Here's how the part is built. I have some questions about the finished solid (model axes, mm). A direction names the side the tool comes from. Give positions to 0.01 mm unless a question says otherwise; leave off trailing zeros. Order: outer loops, then holes, each group sorted by start corner. A loop starts at its lowest first (then second) coordinate and runs counter-clockwise, first axis right, second up.
from build123d import *

# Parameters (mm, degrees)
PAD_DEPTH    = 16
POCKET_DEPTH = 1


with BuildPart() as part:
    # Sketch → Pad (new body)
    with BuildSketch(Plane.XY):
        Polygon((0, 413.879036), (0, 490), (460, 490), (460, 0), (0, 0), align=None)
    extrude(amount=-PAD_DEPTH)

    # Sketch002 (on Face7 of Pad) → Pocket (cut)
    with BuildSketch(Plane(origin=(0, 0, -16), x_dir=(1, 0, 0), z_dir=(0, 0, -1))):
        Polygon((0, 0), (0, -71.973152), (460, 0), align=None)
    extrude(amount=-POCKET_DEPTH, mode=Mode.SUBTRACT)


solid = part.part
Q1. For faces 1 (the face through (0, 248, -8)), 2 (the face through (176, 27, -15)), which set-ups out of +Z, -Z, +X, -X, +Y, -Y let a thin tool reach every point of the face, with its end or its side?
Filled sheet:
face 1: +Z, -Z, -X, +Y, -Y
face 2: -Z, -X, -Y
Q2. I'm going to push a flat-ended pin straight in: P1, Ø1, axis at y = 263.5, z = -4, coming from the -X side. Where does the tip first touch, or does it pass through?
Filled sheet:
P1: stops at x = 0
Q3. If we section it at A-A on y = 53: List the corners of the cut face in (x, z) for me, plus the area to 3 significant figures.
Filled sheet:
outline: (0, -15) - (121.26, -15) - (121.26, -16) - (460, -16) - (460, 0) - (0, 0) - close
area: 7,240 mm2
